from build123d import *

# Parameters (mm, degrees)
F1_DEPTH = 6
F2_R     = 1.5
F3_DEPTH = 6.001
F4_R     = 1.5
F5_DEPTH = 6.001


with BuildPart() as f1:
    # F0 (on Front) → F1 (new body)
    with BuildSketch(Plane.XZ):
        with BuildLine():
            ThreePointArc((0, 8), (-4, 4), (0, 0))
            Line((0, 0), (50, 0))
            ThreePointArc((50, 0), (54, 4), (50, 8))
            Line((50, 8), (0, 8))
        make_face()
    extrude(amount=F1_DEPTH)

    # F2 (on face) → F3 (cut, through all)
    with BuildSketch(Plane.XZ.offset(6)):
        with Locations((0, 4)):
            Circle(F2_R)
    extrude(amount=-F3_DEPTH, mode=Mode.SUBTRACT)

    # F4 (on face) → F5 (cut, through all)
    with BuildSketch(Plane.XZ.offset(6)):
        with Locations((50, 4)):
            Circle(F4_R)
    extrude(amount=-F5_DEPTH, mode=Mode.SUBTRACT)


solid = f1.part
Model file for the job. Use its own axes, mm. Give positions to 0.01 mm unless a question says otherwise; leave off trailing zeros. Order: outer loops, then holes, each group sorted by start corner. A loop starts at its lowest first (then second) coordinate and runs counter-clockwise, first axis right, second up. Notation, with made-up numbers: (33.5, 87.25) - (60.5, 87.25) arc R16 ccw to (60.5, 97.25) - close; hole circle Ø10 at (80.25, 12). An arc over 180 degrees is marked (long way). Write item = value, one per line. Start each with the question number.
1. Two-plate mould, pull along X, no slides. Class faces 1 (the flat face through (25, -3, 8)), 2 (the cylindrical face through (54, -3, 4)), 3 (the cylindrical face through (0.806, -3.042, 5.265)): pulls with the +X half, pulls with the -X half, needs draft (parallel to the pull), parting line crosses it, or undercut.
2. Cut at A-A, the plane z = 4. List the corners of the cut face in (x, y).
3. Probe line 1 along X through (y, z) = (-0.7, 5); line 2 along X through (y, z) = (-5.45, 4.5); line 3 along Z through (x, y) = (0, -3.2). List the from-to ranges inside material, lowest first.
4. Cut at C-C, the plane z = 7.25. List the corners of the cut face in (x, y).
5. Drop flat-ended pins along their axis: P1, Ø4, axis at x = 11, z = 5, coming from the +Y side; P2, Ø1.5, axis at y = -3.5, z = 7, coming from the -X side. Give the stop position or say it passes through.
6. Cut at B-B, the plane y = -0.6. List the corners of the cut face in (x, z).
Taken from the geometry:
q1.face_1 = needs draft
q1.face_2 = pulls with the +X half
q1.face_3 = undercut
q2.outline = (-4, -6) - (-1.5, -6) - (-1.5, 0) - (-4, 0) - close; (1.5, -6) - (48.5, -6) - (48.5, 0) - (1.5, 0) - close; (51.5, -6) - (54, -6) - (54, 0) - (51.5, 0) - close
q3.line_1 = -3.87 to -1.12, 1.12 to 48.88, 51.12 to 53.87
q3.line_2 = -3.97 to -1.41, 1.41 to 48.59, 51.41 to 53.97
q3.line_3 = 0 to 2.5, 5.5 to 8
q4.outline = (-2.33, -6) - (52.33, -6) - (52.33, 0) - (-2.33, 0) - close
q5.P1 = 0
q5.P2 = -3.31
q6.outline = (0, 0) - (50, 0) arc R4 ccw to (50, 8) - (0, 8) arc R4 ccw to start; hole circle Ø3 at (0, 4); hole circle Ø3 at (50, 4)
